The listing builds one solid part. Answer for the finished solid, in the listing's coordinates (mm). Face numbers are marked on the shaded views. A direction names the side the tool comes from. Give positions to 0.01 mm unless a question says otherwise; leave off trailing zeros. Write each loop counter-clockwise with the first axis right and the second up, starting at its lowest first coordinate (ties: lowest second). Pieces come first, ordered by that corner, then holes. Notation, with made-up numbers: M 18.25,1 L 70.25,1 A22 ccw 70.25,18 Z; hole C 22,30.5 d8. An arc over 180 degrees is marked long. Return JSON: item names as keys, results as strings.
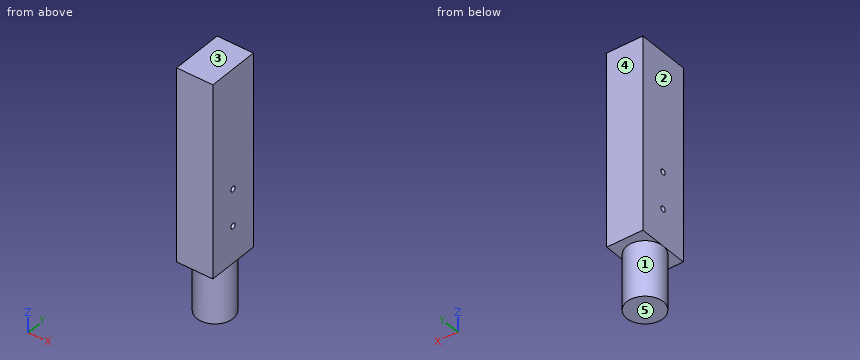
from build123d import *

# Parameters (mm, degrees)
SKETCH1_W           = 19.59343046
SKETCH1_H           = 28.33511482
BOSS_EXTRUDE1_DEPTH = 104.84505691
SKETCH2_R           = 9.79671523
BOSS_EXTRUDE2_DEPTH = 30
SKETCH3_R           = 1.5
CUT_EXTRUDE1_DEPTH  = 111.359717323


with BuildPart() as part:
    # Sketch1 → Boss-Extrude1 (new body)
    with BuildSketch(Plane.XY):
        with Locations((9.79671523, 14.16755741)):
            Rectangle(SKETCH1_W, SKETCH1_H)
    extrude(amount=BOSS_EXTRUDE1_DEPTH)

    # Sketch2 → Boss-Extrude2 (add)
    with BuildSketch(Plane(origin=(0, 0, 0), x_dir=(-1, 0, 0), z_dir=(0, 0, -1))):
        with Locations((-9.79671523, 14.16755741)):
            Circle(SKETCH2_R)
    extrude(amount=BOSS_EXTRUDE2_DEPTH)

    # Sketch3 → Cut-Extrude1 (cut, through all)
    with BuildSketch(Plane(origin=(19.59343046, 0, 0), x_dir=(0, 0, -1), z_dir=(1, 0, 0))):
        with Locations((-20, 14.16755741)):
            Circle(SKETCH3_R)
        with Locations((-40, 14.16755741)):
            Circle(SKETCH3_R)
    extrude(amount=-CUT_EXTRUDE1_DEPTH, mode=Mode.SUBTRACT)


solid = part.part
Item 1: A cutting plane is placed at D-D, the plane z = -10. Write down the section's boundary in (x, y), plus the area to 3 significant figures.
Geometry results:
{"outline": "C 9.8,14.17 d19.59", "area": "302 mm2"}
Item 2: A cutting plane is placed at C-C, the plane y = 19. Write down the section's boundary in (x, z).
Geometry results:
{"outline": "M 0,0 L 1.27,0 L 1.27,-30 L 18.32,-30 L 18.32,0 L 19.59,0 L 19.59,104.85 L 0,104.85 Z"}
Item 3: A cutting plane is placed at B-B, the plane x = 15. Write down the section's boundary in (y, z), plus the area to 3 significant figures.
Geometry results:
{"outline": "M 0,0 L 5.87,0 L 5.87,-30 L 22.47,-30 L 22.47,0 L 28.34,0 L 28.34,104.85 L 0,104.85 Z; hole C 14.17,20 d3; hole C 14.17,40 d3", "area": "3,450 mm2"}
Item 4: Which of the six approach directions +Z, -Z, +X, -X, +Y, -Y give full straight-line access (tool end or side, diameter ignored) to the marked faces 1 and 2?
Geometry results:
{"face 1": "-Z", "face 2": "+Z, -Z, -X, +Y, -Y"}
Item 5: Given pin 1 Ø4 at (y, z) = (14.17, 40) entering from -X; pin 2 Ø1.8 at (y, z) = (14.17, 20) entering from -X; pin 3 Ø12 at (y, z) = (22, -7) entering from +X, each flat-ended and moving along its own axis, determine where each tip first touches the part or whether it passes through.
Geometry results:
{"pin 1": "stops at x = 0", "pin 2": "passes through", "pin 3": "stops at x = 19.42"}
Item 6: Find the intervals of material crossed by line 1 (Y direction, x = 11.5, z = 20); line 2 (Z direction, x = 16, y = 22.5); line 3 (Z direction, x = 15, y = 13.5), in increasing order.
Geometry results:
{"line 1": "y = 0 to 12.67, 15.67 to 28.34", "line 2": "z = 0 to 104.85", "line 3": "z = -30 to 18.66, 21.34 to 38.66, 41.34 to 104.85"}
Item 7: Determine the mould class of the marked faces 3, 4 and 5 for opening direction Z: +Z half, -Z half, draft (parallel to the pull), parting line (faces both ways), or undercut.
Geometry results:
{"face 3": "+Z half", "face 4": "draft", "face 5": "-Z half"}
Item 8: A cutting plane is placed at A-A, the plane z = 20. Write down the section's boundary in (x, y), plus the area to 3 significant figures.
Geometry results:
{"outline": "M 0,0 L 19.59,0 L 19.59,12.67 L 0,12.67 Z; M 0,15.67 L 19.59,15.67 L 19.59,28.34 L 0,28.34 Z", "area": "496 mm2"}
